Model file for the job. Use its own axes, mm. Face numbers are marked on the shaded views. A direction names the side the tool comes from. Round coordinates to 2 decimals unless told otherwise and drop trailing zeros. Order: outer loops, then holes, each group sorted by start corner. A loop starts at its lowest first (then second) coordinate and runs counter-clockwise, first axis right, second up. Notation, with made-up numbers: (35.5, 86) -> (82.5, 86) arc R20 cw to (82.5, 104) -> close; hole circle Ø3 at (0, -1). An arc over 180 degrees is marked (long way). Use CSV: the item, a comma, the result in double quotes.
Autodesk Inventor part; units mm, degrees
ref_plane "YZ Plane" through (0, 0, 0) normal (1, 0, 0) x (0, 1, 0)
ref_plane "XZ Plane" through (0, 0, 0) normal (0, 1, 0) x (-1, 0, 0)
ref_plane "XY Plane" through (0, 0, 0) normal (0, 0, 1) x (1, 0, 0)
sketch "Boceto1" plane through (0, 0, 0) normal (0, 0, 1) x (1, 0, 0)
  line L0 (-15, 45) -> (15, 45)
  line L1 (15, 45) -> (15, -45)
  line L2 (15, -45) -> (-15, -45)
  line L3 (-15, -45) -> (-15, 45)
  line L4 (-15, 45) -> (15, -45) construction
  line L5 (15, 45) -> (-15, -45) construction
  point P0 (0, 0)
  dimension "d0" = 30
  dimension "d1" = 90
extrude "Extrusión1" add sketch "Boceto1" along normal blind 10
sketch "Boceto2" plane through (0, 0, 10) normal (0, 0, 1) x (1, 0, 0)
  line L0 (15, 45) -> (15, -45)
  line L1 (5, 30) -> (5, 20)
  line L2 (-5, 30) -> (5, 30)
  line L3 (5, 20) -> (-5, 30) construction
  line L4 (5, 20) -> (-5, 20)
  line L5 (-5, 20) -> (5, 30) construction
  line L6 (-5, 20) -> (-5, 30)
  line L7 (24, 0) -> (9, 0)
  line L8 (-15, -45) -> (15, -45)
  line L9 (5, 25) -> (5.4102, 25)
  circle A0 centre (-3.25, 21.75) radius 1.75
  circle A1 centre (3.25, 28.25) radius 1.75
  line L10 (5, -20) -> (-5, -20)
  circle A2 centre (-3.25, -21.75) radius 1.75
  line L11 (5, -25) -> (5.4102, -25)
  line L12 (5, -30) -> (5, -20)
  line L13 (-5, -30) -> (5, -30)
  line L14 (5, -20) -> (-5, -30) construction
  line L15 (-5, -20) -> (5, -30) construction
  line L16 (-5, -20) -> (-5, -30)
  circle A3 centre (3.25, -28.25) radius 1.75
  line L17 (-15, -45) -> (-15, 45)
  line L18 (15, -45) -> (15, 45)
  line L19 (-15, -45) -> (15, -45)
  line L20 (-15, 45) -> (15, 45)
  line L21 (-3.25, 28.25) -> (3.25, 21.75)
  line L22 (-3.25, 21.75) -> (3.25, 28.25)
  point P0 (0, 0)
  point P1 (-113, 215)
  point P2 (-5, 25)
  point P3 (-3.25, -21.75)
  point P4 (3.25, -28.25)
  point P5 (-143, 115)
  point P6 (-3.25, -21.75)
  point P7 (-5, -25)
  point P8 (3.25, -28.25)
  point P9 (0, 25)
  point P10 (0, -25)
  dimension "d4" = 1.75
  dimension "d5" = 1.75
  dimension "d6" = 1.75
  dimension "d7" = 1.75
  dimension "d8" = 10
  dimension "d9" = 10
  dimension "d10" = 10
  dimension "d11" = 15
  dimension "d12" = 0
  dimension "d13" = 30
  dimension "d14" = 0
  dimension "d15" = 90
  dimension "d16" = 15
hole "Agujero1" at (3.25, 28.25, 10) at (-3.25, 21.75, 10) at (-3.25, -21.75, 10) at (3.25, -28.25, 10) direction (0, 0, -1) diameter 3.5 end through all
sketch "Boceto3" plane through (-15, -45, 0) normal (-1, 0, 0) x (0, 0, 1)
  line L0 (0, 0) -> (0, 90)
  line L1 (0, 90) -> (20, 90)
  line L2 (20, 90) -> (20, 0)
  line L3 (20, 0) -> (0, 0)
  line L4 (0, 0) -> (0, 90)
  point P0 (0, 45)
  dimension "d24" = 20
  dimension "d25" = 90
extrude "Extrusión2" add sketch "Boceto3" along normal blind 10
sketch "Boceto4" plane through (-25, -45, 0) normal (-1, 0, 0) x (0, 0, 1)
  line L0 (20, 90) -> (10, 90)
  line L1 (10, 0) -> (10, 90)
  line L2 (20, 90) -> (10, 90)
  line L3 (10, 90) -> (10, 0)
  line L4 (10, 0) -> (20, 0)
  line L5 (20, 0) -> (20, 90)
  point P0 (0, 45)
extrude "Extrusión3" add sketch "Boceto4" along normal blind 30
sketch "Boceto5" plane through (-15, -45, 20) normal (0, 0, 1) x (1, 0, 0)
  line L0 (-40, 0) -> (-70, 90)
  line L1 (-70, 90) -> (-40, 0)
  line L2 (-20, 75) -> (-20, 65)
  line L3 (-30, 75) -> (-20, 75)
  line L4 (-20, 65) -> (-30, 75) construction
  line L5 (-20, 65) -> (-30, 65)
  line L6 (-30, 65) -> (-20, 75) construction
  circle A0 centre (-28.25, 66.75) radius 1.75
  line L7 (-30, 65) -> (-30, 75)
  circle A1 centre (-21.75, 73.25) radius 1.75
  line L8 (-40, -20) -> (-40, 90)
  line L9 (-55, 45) -> (-143, 45)
  line L10 (-20, 25) -> (-30, 25)
  circle A2 centre (-28.25, 23.25) radius 1.75
  line L11 (-20, 15) -> (-20, 25)
  line L12 (-20, 25) -> (-30, 15) construction
  line L13 (-30, 25) -> (-20, 15) construction
  line L14 (-30, 25) -> (-30, 15)
  line L15 (-30, 15) -> (-20, 15)
  circle A3 centre (-21.75, 16.75) radius 1.75
  line L16 (-70, 0) -> (-40, 0)
  line L17 (0, 0) -> (-40, 0)
  line L18 (-40, 90) -> (-70, 90)
  line L19 (-40, 0) -> (-40, 90)
  point P0 (15, 45)
  point P1 (-30, 70)
  point P2 (-20, 70)
  point P3 (-20, 20)
  point P4 (-30, 20)
  point P5 (-55, 0)
  point P6 (-55, 90)
  dimension "d30" = 3.5
  dimension "d31" = 1.75
  dimension "d32" = 1.75
  dimension "d33" = 1.75
  dimension "d34" = 1.75
  dimension "d35" = 10
  dimension "d36" = 10
  dimension "d38" = 10
  dimension "d39" = -41.1096
  dimension "d40" = 15
  dimension "d41" = 0
  dimension "d42" = 15
  dimension "d43" = 90
  dimension "d45" = 0
hole "Agujero2" at (-36.75, 28.25, 20) at (-43.25, 21.75, 20) at (-43.25, -21.75, 20) at (-36.75, -28.25, 20) direction (0, 0, -1) diameter 3.5 end through all
sketch "Boceto6" plane through (-15, -45, 20) normal (0, 0, 1) x (1, 0, 0)
  line L0 (-10, 0) -> (-40, 0)
  line L1 (-40, 0) -> (60, 0)
  line L2 (60, 0) -> (60, -20)
  line L3 (60, -20) -> (-40, -20)
  line L4 (-40, -20) -> (-40, 0)
  point P0 (15, 45)
  dimension "d53" = 20
extrude "Extrusión4" add sketch "Boceto6" against normal blind 100
mirror "Simetría1" about plane through (-5, -55, -80) normal (0, 0, -1) of "Extrusión1", "Agujero1", "Extrusión2", "Agujero2", "Extrusión3", "Extrusión4"
ref_plane "Plano de trabajo2" through (45, -65, -80) normal (0, 0, -1) x (-1, 0, 0)
sketch "Boceto7" plane through (-15, -45, 20) normal (0, 1, 0) x (1, 0, 0)
  line L0 (30, 115) -> (30, 85)
  circle A0 centre (35, 90) radius 1.75
  line L1 (30, 85) -> (40, 85)
  line L2 (35, 110) -> (35, 90)
  circle A1 centre (35, 110) radius 1.75
  line L3 (40, 115) -> (30, 85) construction
  line L4 (40, 115) -> (30, 115)
  line L5 (30, 115) -> (40, 85) construction
  line L6 (40, 85) -> (40, 115)
  line L7 (60, 0) -> (60, 200)
  line L8 (-40, 0) -> (60, 0)
  line L9 (10, 0) -> (10, 134.4524)
  line L10 (-10, 115) -> (-10, 85)
  circle A2 centre (-15, 110) radius 1.75
  line L11 (-20, 115) -> (-10, 115)
  circle A3 centre (-15, 90) radius 1.75
  line L12 (-10, 85) -> (-20, 85)
  line L13 (-20, 115) -> (-10, 85) construction
  line L14 (-10, 115) -> (-20, 85) construction
  line L15 (-20, 85) -> (-20, 115)
  line L16 (-15, 110) -> (-15, 90)
  point P0 (15, 20)
  point P1 (189.1833, 40)
  point P2 (35, 115)
  point P3 (-85.8367, 100)
  point P4 (235.02, 100)
  point P5 (-15, 115)
  dimension "d56" = 5
  dimension "d57" = 5
  dimension "d58" = 3.5
  dimension "d59" = 5
  dimension "d60" = 5
  dimension "d61" = 10
  dimension "d62" = 30
  dimension "d64" = 20
hole "Agujero3" at (-30, -45, -90) at (-30, -45, -70) at (20, -45, -90) at (20, -45, -70) direction (0, -1, 0) diameter 3.5 end through all
properties part number "container_mid"
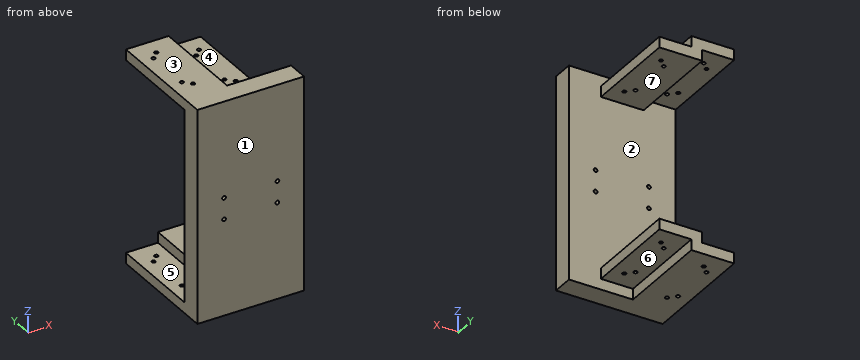
Q1. Pin check, flat tips, straight feed: pin 1 (3 mm diameter, centred on x = 3.25, y = 28.25, fed in from +Z); pin 2 (3 mm diameter, centred on y = -14.5, z = -175.5, fed in from +X); pin 3 (12 mm diameter, centred on x = -16, z = -8, fed in from +Y); pin 4 (8 mm diameter, centred on y = 8, z = -167, fed in from +X). Stop position of each tip, or through.
From the geometry:
pin 1,"passes through"
pin 2,"stops at x = -15"
pin 3,"stops at y = -45"
pin 4,"stops at x = 15"
Q2. Mould opens along Z. For the marked faces 1, 2 and 3 say: +Z half, -Z half, draft (parallel to the pull), parting line (faces both ways), or undercut.
From the geometry:
face 1,"draft"
face 2,"undercut"
face 3,"+Z half"
Q3. Cut at A-A (x = 11). Give the cut face in (y, z), plus the area to 3 significant figures.
From the geometry:
outline,"(-65, -180) -> (-45, -180) -> (-45, -170) -> (45, -170) -> (45, -160) -> (-45, -160) -> (-45, 0) -> (45, 0) -> (45, 10) -> (-45, 10) -> (-45, 20) -> (-65, 20) -> close"
area,"5,800 mm²"
Q4. Which spindle directions (+Z, -Z, +X, -X, +Y, -Y) get a long thin tool onto all of the face, cutting with end or side? Do the marked faces 4, 5, 6 and 7. Say none if no direction does.
From the geometry:
face 4,"+Z, +X, +Y"
face 5,"-X, +Y"
face 6,"-Z, +X, +Y"
face 7,"+X, -X, +Y"
Q5. Cut at C-C (x = 38.5). Give the cut face in (y, z), plus the area to 3 significant figures.
From the geometry:
outline,"(-65, -180) -> (-45, -180) -> (-45, 20) -> (-65, 20) -> close"
area,"4,000 mm²"
Q6. Cut at B-B (z = -151). Give the cut face in (x, y), plus the area to 3 significant figures.
From the geometry:
outline,"(-55, -65) -> (45, -65) -> (45, -45) -> (-55, -45) -> close"
area,"2,000 mm²"
Q7. Probe line 1 along X through (y, z) = (-53.5, -70); line 2 along Z through (x, y) = (20, -51); line 3 along Y through (x, z) = (-43.25, 16). List the from-to ranges inside material, lowest first.
From the geometry:
line 1,"x = -55 to -31.75, -28.25 to 18.25, 21.75 to 45"
line 2,"z = -180 to -91.75, -88.25 to -71.75, -68.25 to 20"
line 3,"y = -65 to -23.5, -20 to 20, 23.5 to 45"
